from build123d import *

# Parameters (mm, degrees)
MODEL_W            = 64.9
MODEL_H            = 84.15
MODEL_R            = 1.45
BOSS_EXTRU_2_DEPTH = 3
CONG_1_R           = 1
CONG_2_R           = 1
CONG_4_R           = 1
CONG_5_R           = 1


with BuildPart() as part:
    # Model → Boss.-Extru.2 (new body)
    with BuildSketch(Plane.XY):
        with Locations((19.8375, -9.525)):
            Rectangle(MODEL_W, MODEL_H)
        with Locations((-7.6125, 27.55)):
            Circle(MODEL_R, mode=Mode.SUBTRACT)
        with Locations((47.2875, 27.55)):
            Circle(MODEL_R, mode=Mode.SUBTRACT)
        with Locations((47.2875, -46.6)):
            Circle(MODEL_R, mode=Mode.SUBTRACT)
        with Locations((-7.6125, -46.6)):
            Circle(MODEL_R, mode=Mode.SUBTRACT)
        with BuildLine():
            Line((3.025, -2.525), (16.025, -2.525))
            ThreePointArc((16.025, -2.525), (16.378553391, -2.671446609), (16.525, -3.025))
            Line((16.525, -3.025), (16.525, -16.025))
            ThreePointArc((16.525, -16.025), (16.378553391, -16.378553391), (16.025, -16.525))
            Line((16.025, -16.525), (3.025, -16.525))
            ThreePointArc((3.025, -16.525), (2.671446609, -16.378553391), (2.525, -16.025))
            Line((2.525, -16.025), (2.525, -3.025))
            ThreePointArc((2.525, -3.025), (2.671446609, -2.671446609), (3.025, -2.525))
        make_face(mode=Mode.SUBTRACT)
        with BuildLine():
            Line((23.65, -2.525), (36.65, -2.525))
            ThreePointArc((36.65, -2.525), (37.003553391, -2.671446609), (37.15, -3.025))
            Line((37.15, -3.025), (37.15, -16.025))
            ThreePointArc((37.15, -16.025), (37.003553391, -16.378553391), (36.65, -16.525))
            Line((36.65, -16.525), (23.65, -16.525))
            ThreePointArc((23.65, -16.525), (23.296446609, -16.378553391), (23.15, -16.025))
            Line((23.15, -16.025), (23.15, -3.025))
            ThreePointArc((23.15, -3.025), (23.296446609, -2.671446609), (23.65, -2.525))
        make_face(mode=Mode.SUBTRACT)
        with BuildLine():
            Line((3.025, -21.575), (16.025, -21.575))
            ThreePointArc((16.025, -21.575), (16.378553391, -21.721446609), (16.525, -22.075))
            Line((16.525, -22.075), (16.525, -35.075))
            ThreePointArc((16.525, -35.075), (16.378553391, -35.428553391), (16.025, -35.575))
            Line((16.025, -35.575), (3.025, -35.575))
            ThreePointArc((3.025, -35.575), (2.671446609, -35.428553391), (2.525, -35.075))
            Line((2.525, -35.075), (2.525, -22.075))
            ThreePointArc((2.525, -22.075), (2.671446609, -21.721446609), (3.025, -21.575))
        make_face(mode=Mode.SUBTRACT)
        with BuildLine():
            Line((23.65, -21.575), (36.65, -21.575))
            ThreePointArc((36.65, -21.575), (37.003553391, -21.721446609), (37.15, -22.075))
            Line((37.15, -22.075), (37.15, -35.075))
            ThreePointArc((37.15, -35.075), (37.003553391, -35.428553391), (36.65, -35.575))
            Line((36.65, -35.575), (23.65, -35.575))
            ThreePointArc((23.65, -35.575), (23.296446609, -35.428553391), (23.15, -35.075))
            Line((23.15, -35.075), (23.15, -22.075))
            ThreePointArc((23.15, -22.075), (23.296446609, -21.721446609), (23.65, -21.575))
        make_face(mode=Mode.SUBTRACT)
    extrude(amount=BOSS_EXTRU_2_DEPTH)

    # Congé1
    cong_1_edges = [part.edges().sort_by_distance(p)[0] for p in [
        (-12.6125, -9.525, 3),
    ]]
    fillet(cong_1_edges, radius=CONG_1_R)

    # Congé2
    cong_2_edges = [part.edges().sort_by_distance(p)[0] for p in [
        (52.2875, -9.525, 3),
    ]]
    fillet(cong_2_edges, radius=CONG_2_R)

    # Congé4
    cong_4_edges = [part.edges().sort_by_distance(p)[0] for p in [
        (19.8375, -51.6, 3),
        (-12.6125, -51.6, 1),
        (-12.319606781, -51.6, 2.707106781),
        (52.2875, -51.6, 1),
        (51.994606781, -51.6, 2.707106781),
    ]]
    fillet(cong_4_edges, radius=CONG_4_R)

    # Congé5
    cong_5_edges = [part.edges().sort_by_distance(p)[0] for p in [
        (-12.6125, 32.55, 1),
        (-12.319606781, 32.55, 2.707106781),
        (19.8375, 32.55, 3),
        (52.2875, 32.55, 1),
        (51.994606781, 32.55, 2.707106781),
    ]]
    fillet(cong_5_edges, radius=CONG_5_R)


solid = part.part
Geometry check sheet. Reference: the model listing, model coordinates, mm. A direction names the side the tool comes from. Round coordinates to 2 decimals unless told otherwise and drop trailing zeros. Order: outer loops, then holes, each group sorted by start corner. A loop starts at its lowest first (then second) coordinate and runs counter-clockwise, first axis right, second up. Notation, with made-up numbers: M -34.5,31 L -0.5,31 A17 cw -0.5,54 Z; hole C 33.25,34 d11. An arc over 180 degrees is marked long. Write each question's results on one line, items separated by ' | '. Start each with the question number.
1. Cross-section at B-B on x = 28.5. Record the boundary of the cut face in (y, z) (3 decimals), plus the area to 3 significant figures.
2. Draft check along Y on faces 3 (the face through (19, 32.55, 1)), 4 (the face through (19, -9, 0)), 5 (the face through (16.525, -9, 1)). Enter one of: pulls with the +Y half, pulls with the -Y half, needs draft (parallel to the pull), parting line crosses it, or undercut.
3. Set-up check for faces 1 (the face through (37.15, -9, 1)), 2 (the face through (-12.613, -10, 1)): record each of +Z, -Z, +X, -X, +Y, -Y from which the full face is reachable in a straight line by a thin tool's end or side.
4. Material ranges on L1, parallel to Y at x = 32.5, z = 0.45 (3 decimals); L2, parallel to Y at x = 25.5, z = 2.05 (3 decimals); L3, parallel to X at y = 17, z = 2.1, recorded low to high. Write a range as from..to.
5. Cross-section at C-C on z = 2.45. Give the number of separate pieces and of enclosed holes in the cut face, plus the area to 3 significant figures.
6. Cross-section at A-A on y = 27.55. Record the boundary of the cut face in (x, z), plus the area to 3 significant figures.
Resolved:
1) outline: M -51.6,0 L -35.575,0 L -35.575,3 L -50.6,3 A1 ccw -51.6,2 Z; M -21.575,0 L -16.525,0 L -16.525,3 L -21.575,3 Z; M -2.525,0 L 32.55,0 L 32.55,2 A1 ccw 31.55,3 L -2.525,3 Z | area: 168 mm2
2) face 3: pulls with the +Y half | face 4: needs draft | face 5: undercut
3) face 1: +Z, -Z | face 2: +Z, -Z, -X, +Y, -Y
4) L1: -51.6..-35.575, -21.575..-16.525, -2.525..32.55 | L2: -51.599..-35.575, -21.575..-16.525, -2.525..32.549 | L3: -12.61..52.28
5) separate pieces: 1 | enclosed holes: 8 | area: 4,620 mm2
6) outline: M -12.61,0 L -9.06,0 L -9.06,3 L -11.61,3 A1 ccw -12.61,2 Z; M -6.16,0 L 45.84,0 L 45.84,3 L -6.16,3 Z; M 48.74,0 L 52.29,0 L 52.29,2 A1 ccw 51.29,3 L 48.74,3 Z | area: 177 mm2
